from build123d import *

# Parameters (mm, degrees)
ESQUISSE1_R        = 3
ESQUISSE1_R_2      = 0.75
BOSS_EXTRU_1_DEPTH = 3


with BuildPart() as part:
    # Esquisse1 → Boss.-Extru.1 (new body)
    with BuildSketch(Plane.XY):
        with BuildLine():
            Line((0, -5.9), (-20, -5.9))
            ThreePointArc((-20, -5.9), (-25.9, 0), (-20, 5.9))
            Line((-20, 5.9), (0, 5.9))
            ThreePointArc((0, 5.9), (5.9, 0), (0, -5.9))
        make_face()
        Circle(ESQUISSE1_R, mode=Mode.SUBTRACT)
        with Locations((-21, 0)):
            Circle(ESQUISSE1_R_2, mode=Mode.SUBTRACT)
        with Locations((-18, 0)):
            Circle(ESQUISSE1_R_2, mode=Mode.SUBTRACT)
        with Locations((-15, 0)):
            Circle(ESQUISSE1_R_2, mode=Mode.SUBTRACT)
        with Locations((-12, 0)):
            Circle(ESQUISSE1_R_2, mode=Mode.SUBTRACT)
        with Locations((-9, 0)):
            Circle(ESQUISSE1_R_2, mode=Mode.SUBTRACT)
    extrude(amount=-BOSS_EXTRU_1_DEPTH)

    # Esquisse2 → Révolution1 (revolve)
    with BuildSketch(Plane(origin=(0, 0, 0), x_dir=(1, 0, 0), z_dir=(0, 1, 0))):
        Polygon((-4.75, 6.2), (-2.75, 6.2), (-2.75, 3), (-1.5, 3), (-1.5, 1.5), (-4.75, 1.5), align=None)
    revolve(axis=Axis((0, 0, -6.2), (0, 0, 1)))


solid = part.part
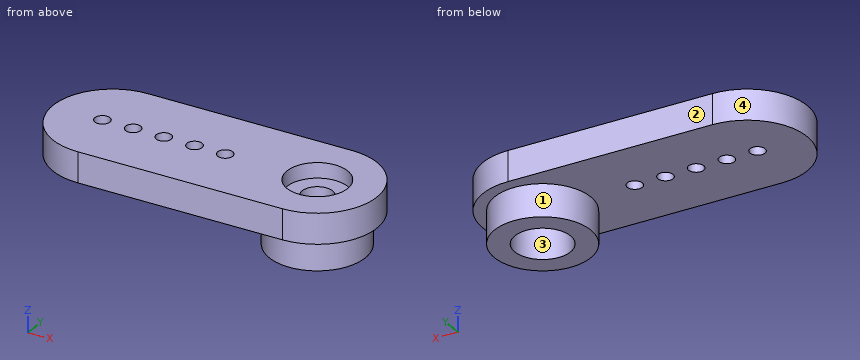
Design review of the part built by this model. Coordinates are the model's own, in mm. Face numbers are marked on the shaded views. Coordinates: 2 decimals unless noted, no trailing zeros. Order: outer loops, then holes, each group sorted by start corner. A loop starts at its lowest first (then second) coordinate and runs counter-clockwise, first axis right, second up. Notation, with made-up numbers: (34.5, 28) - (83.5, 28) arc R29 cw to (83.5, 48) - close; hole circle Ø7 at (34.25, 40). An arc over 180 degrees is marked (long way). Put each result on its own line as item: value.
1) Insertion check: P1, Ø2, axis at y = -2.5, z = -5.5, coming from the +X side; P2, Ø0.9, axis at x = -21, y = 0, coming from the +Z side; P3, Ø2, axis at x = -15, y = 0, coming from the -Z side. Each pin has a flat end and moves straight along its axis. Give the tip position at first contact, or say it passes through.
Response values:
P1: stops at x = 4.51
P2: passes through
P3: stops at z = -3
2) Take a section at C-C, the plane z = -5.25. Give the boundary of the cut face in (x, y).
Response values:
outline: circle Ø9.5 at (0, 0); hole circle Ø5.5 at (0, 0)
3) Take a section at B-B, the plane z = -0.5. Give the boundary of the cut face in (x, y), and give its area (3 significant figures).
Response values:
outline: (-20, -5.9) - (0, -5.9) arc R5.9 ccw to (0, 5.9) - (-20, 5.9) arc R5.9 ccw to start; hole circle Ø1.5 at (-21, 0); hole circle Ø1.5 at (-18, 0); hole circle Ø1.5 at (-15, 0); hole circle Ø1.5 at (-12, 0); hole circle Ø1.5 at (-9, 0); hole circle Ø6 at (0, 0)
area: 308 mm²
4) Take a section at A-A, the plane x = -12. Give the boundary of the cut face in (y, z), and give its area (3 significant figures).
Response values:
outline: (-5.9, -3) - (-0.75, -3) - (-0.75, 0) - (-5.9, 0) - close; (0.75, -3) - (5.9, -3) - (5.9, 0) - (0.75, 0) - close
area: 30.9 mm²
5) Take a section at D-D, the plane x = 2. Give the boundary of the cut face in (y, z).
Response values:
outline: (-5.55, -3) - (-4.31, -3) - (-4.31, -6.2) - (-1.89, -6.2) - (-1.89, -3) - (1.89, -3) - (1.89, -6.2) - (4.31, -6.2) - (4.31, -3) - (5.55, -3) - (5.55, 0) - (2.24, 0) - (2.24, -1.5) - (-2.24, -1.5) - (-2.24, 0) - (-5.55, 0) - close
6) Wall thickness on L1, parallel to X at y = 0, z = -4.65; L2, parallel to Z at x = -15, y = -5; L3, parallel to Y at x = -9, z = -1.6: over which ranges is each line inside the solid? List them lowest first. Write a range as from..to.
Response values:
L1: x = -4.75..-2.75, 2.75..4.75
L2: z = -3..0
L3: y = -5.9..-0.75, 0.75..5.9
7) The part is to be moulded in two halves that separate along X. For the marked faces 1, 2, 3 and 4, say which applies: released by +X, released by -X, zero draft, split by the parting line, or undercut.
Response values:
face 1: split by the parting line
face 2: zero draft
face 3: undercut
face 4: released by -X
